Build history of the part. All positions in model axes, mm. Give positions to 0.01 mm unless a question says otherwise; leave off trailing zeros. Write each loop counter-clockwise with the first axis right and the second up, starting at its lowest first coordinate (ties: lowest second). Pieces come first, ordered by that corner, then holes.
Autodesk Inventor part; units mm, degrees
ref_plane "YZ Plane" through (0, 0, 0) normal (1, 0, 0) x (0, 1, 0)
ref_plane "XZ Plane" through (0, 0, 0) normal (0, 1, 0) x (-1, 0, 0)
ref_plane "XY Plane" through (0, 0, 0) normal (0, 0, 1) x (1, 0, 0)
sketch "Sketch1" plane through (0, 0, 0) normal (0, 0, 1) x (1, 0, 0)
  line L0 (-38.1609, 0) -> (53.0268, 0) construction
  line L1 (0, -35.8177) -> (0, 38.9679) construction
  line L2 (0, 0) -> (28.2843, 28.2843) construction
  line L3 (0, 0) -> (40, 0) construction
  line L4 (0, 24.9041) -> (16.9, 24.9041)
  line L5 (16.9, 24.9041) -> (16.9, 21.2841)
  line L6 (16.9, 21.2841) -> (19.092, 19.092)
  line L7 (24.9041, 0) -> (24.9041, 16.9)
  line L8 (24.9041, 16.9) -> (21.2841, 16.9)
  line L9 (21.2841, 16.9) -> (19.092, 19.092)
  line L10 (0, 24.9041) -> (-16.9, 24.9041)
  line L11 (-16.9, 24.9041) -> (-16.9, 21.2841)
  line L12 (-16.9, 21.2841) -> (-19.092, 19.092)
  line L13 (-24.9041, 0) -> (-24.9041, 16.9)
  line L14 (-24.9041, 16.9) -> (-21.2841, 16.9)
  line L15 (-21.2841, 16.9) -> (-19.092, 19.092)
  line L16 (0, -24.9041) -> (16.9, -24.9041)
  line L17 (16.9, -24.9041) -> (16.9, -21.2841)
  line L18 (16.9, -21.2841) -> (19.092, -19.092)
  line L19 (24.9041, 0) -> (24.9041, -16.9)
  line L20 (24.9041, -16.9) -> (21.2841, -16.9)
  line L21 (21.2841, -16.9) -> (19.092, -19.092)
  line L22 (0, -24.9041) -> (-16.9, -24.9041)
  line L23 (-16.9, -24.9041) -> (-16.9, -21.2841)
  line L24 (-16.9, -21.2841) -> (-19.092, -19.092)
  line L25 (-24.9041, 0) -> (-24.9041, -16.9)
  line L26 (-24.9041, -16.9) -> (-21.2841, -16.9)
  line L27 (-21.2841, -16.9) -> (-19.092, -19.092)
  circle A0 centre (0, 0) radius 12.5
  circle A1 centre (-15.5, 15) radius 1.5
  line L28 (-18.5, 18) -> (-12.5, 18) construction
  line L29 (-12.5, 18) -> (-12.5, -12) construction
  line L30 (-12.5, -12) -> (-18.5, -12) construction
  line L31 (-18.5, -12) -> (-18.5, 18) construction
  line L32 (-15.5, 18) -> (-15.5, -12) construction
  circle A2 centre (15.5, -15) radius 1.5
  line L33 (-17.13, 25.1341) -> (0, 25.1341)
  line L34 (0, 25.1341) -> (17.13, 25.1341)
  line L35 (17.13, 25.1341) -> (17.13, 21.3793)
  line L36 (17.13, 21.3793) -> (19.2547, 19.2547)
  line L37 (19.2547, 19.2547) -> (21.3793, 17.13)
  line L38 (21.3793, 17.13) -> (25.1341, 17.13)
  line L39 (25.1341, 17.13) -> (25.1341, 0)
  line L40 (25.1341, 0) -> (25.1341, -17.13)
  line L41 (25.1341, -17.13) -> (21.3793, -17.13)
  line L42 (21.3793, -17.13) -> (19.2547, -19.2547)
  line L43 (19.2547, -19.2547) -> (17.13, -21.3793)
  line L44 (17.13, -21.3793) -> (17.13, -25.1341)
  line L45 (17.13, -25.1341) -> (0, -25.1341)
  line L46 (0, -25.1341) -> (-17.13, -25.1341)
  line L47 (-17.13, -25.1341) -> (-17.13, -21.3793)
  line L48 (-17.13, -21.3793) -> (-19.2547, -19.2547)
  line L49 (-19.2547, -19.2547) -> (-21.3793, -17.13)
  line L50 (-21.3793, -17.13) -> (-25.1341, -17.13)
  line L51 (-25.1341, -17.13) -> (-25.1341, 0)
  line L52 (-25.1341, 0) -> (-25.1341, 17.13)
  line L53 (-25.1341, 17.13) -> (-21.3793, 17.13)
  line L54 (-21.3793, 17.13) -> (-19.2547, 19.2547)
  line L55 (-19.2547, 19.2547) -> (-17.13, 21.3793)
  line L56 (-17.13, 21.3793) -> (-17.13, 25.1341)
  dimension "d0" = 45
  dimension "d1" = 16.9
  dimension "d2" = 3.62
  dimension "d3" = 3.1
  dimension "d4" = 25
  dimension "d5" = 3
  dimension "d11" = 6
  dimension "d12" = 3
  dimension "d14" = 15
  dimension "d15" = 3
  dimension "d16" = 15
  dimension "d17" = 15.5
  dimension "d18" = 15.5
  dimension "d19" = 30
  dimension "d20" = 0.23
extrude "Extrusion1" add sketch "Sketch1" along normal blind 2.5 contours L4 L5 L6 L9 L8 L7 L19 L20 L21 L18 L17 L16 L22 L23 L24 L27 L26 L25 L13 L14 L15 L12 L11 L10 | L33 L34 L35 L36 L37 L38 L39 L40 L41 L42 L43 L44 L45 L46 L47 L48 L49 L50 L51 L52 L53 L54 L55 L56
properties part number "LC_sample_holder_insert"
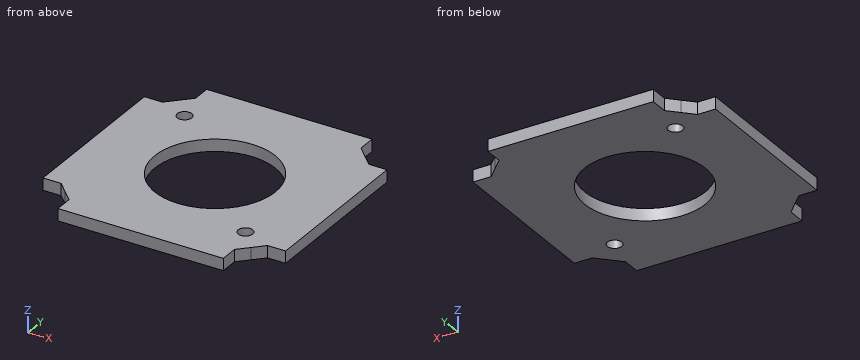
(1) Saw through at B-B, the plane x = 15.5. List the corners of the cut face in (y, z), plus the area to 3 significant figures.
(2) Saw through at D-D, the plane y = -20.5. List the corners of the cut face in (x, z).
(3) Saw through at C-C, the plane z = 1.6. List the corners of the cut face in (x, y).
(4) Drop flat-ended pins along their axis: pin 1 (0.8 mm diameter, centred on x = -23.5, z = 1, fed in from +Y); pin 2 (22.5 mm diameter, centred on x = 0, y = 0, fed in from -Z); pin 3 (0.8 mm diameter, centred on y = -23, z = 1, fed in from +X); pin 4 (1.2 mm diameter, centred on y = 24, z = 0.5, fed in from -X). Give the stop position or say it passes through.
(5) Saw through at A-A, the plane y = 15. List the corners of the cut face in (x, z), plus the area to 3 significant figures.
(6) Probe line 1 (Y direction, x = -15.5, z = 0.55); line 2 (Y direction, x = 15.5, z = 0.95); line 3 (X direction, y = 11, z = 0.7). List the from-to ranges inside material, lowest first.
Computed values:
1. outline: (-25.13, 0) - (-16.5, 0) - (-16.5, 2.5) - (-25.13, 2.5) - close; (-13.5, 0) - (25.13, 0) - (25.13, 2.5) - (-13.5, 2.5) - close
1. area: 118 mm2
2. outline: (-18.01, 0) - (18.01, 0) - (18.01, 2.5) - (-18.01, 2.5) - close
3. outline: (-25.13, -17.13) - (-21.38, -17.13) - (-19.25, -19.25) - (-17.13, -21.38) - (-17.13, -25.13) - (17.13, -25.13) - (17.13, -21.38) - (19.25, -19.25) - (21.38, -17.13) - (25.13, -17.13) - (25.13, 17.13) - (21.38, 17.13) - (19.25, 19.25) - (17.13, 21.38) - (17.13, 25.13) - (-17.13, 25.13) - (-17.13, 21.38) - (-19.25, 19.25) - (-21.38, 17.13) - (-25.13, 17.13) - close; hole circle Ø3 at (-15.5, 15); hole circle Ø25 at (0, 0); hole circle Ø3 at (15.5, -15)
4. pin 1: stops at y = 17.13
4. pin 2: passes through
4. pin 3: stops at x = 17.13
4. pin 4: stops at x = -17.13
5. outline: (-25.13, 0) - (-17, 0) - (-17, 2.5) - (-25.13, 2.5) - close; (-14, 0) - (25.13, 0) - (25.13, 2.5) - (-14, 2.5) - close
5. area: 118 mm2
6. line 1: y = -25.13 to 13.5, 16.5 to 25.13
6. line 2: y = -25.13 to -16.5, -13.5 to 25.13
6. line 3: x = -25.13 to -5.94, 5.94 to 25.13
